Geometry: see drawing. Coordinates: mm, zero at the bounding-box minimum. A direction names the side the tool comes from. Coordinates: 2 decimals unless noted, no trailing zeros. Loops run counter-clockwise (first coordinate to the right, second up) from the corner with the lowest first, then second, coordinate; pieces in that order, holes last. Notation, with made-up numbers: (-27, -30) -> (18, -30) arc R10 cw to (18, -13) -> close; hole circle Ø6 at (43, 20.5). An arc over 180 degrees is marked (long way). Put each result on its own line as item: value. Start each with the question number.
1) Set-up query: the marked faces 1, 2 and 3. Return all of +Z, -Z, +X, -X, +Y, -Y with unobstructed straight access to the full face (end or side cutting, diameter ignored); none if empty.
2) Contact query for flat-ended pins moving along their axis: P1, Ø1, axis at x = 8.5, z = 7.5, coming from the -Y side; P2, Ø0.9, axis at x = 14.5, z = 4, coming from the -Y side; P3, Ø5, axis at x = 30, y = 10, coming from the -Z side. Output: stop coordinate, or through.
3) Cut plane A-A (x = 10). Return the cut outline in (y, z).
4) Cut plane C-C (x = 30). Return the cut outline in (y, z), plus the area to 3 significant figures.
5) Material intervals for L1, parallel to Y at x = 30, z = 3.75; L2, parallel to Y at x = 33, z = 1; L3, parallel to X at y = 30, z = 1.2, sorted ascending.
6) Pull-direction query (Z, two-part tool) for the marked faces 4, 5 and 6; classes: pulls with the +Z half, pulls with the -Z half, needs draft (parallel to the pull), parting line crosses it, or undercut.
7) Cut plane D-D (z = 1.25). Return the cut outline in (x, y), plus the area to 3 significant figures.
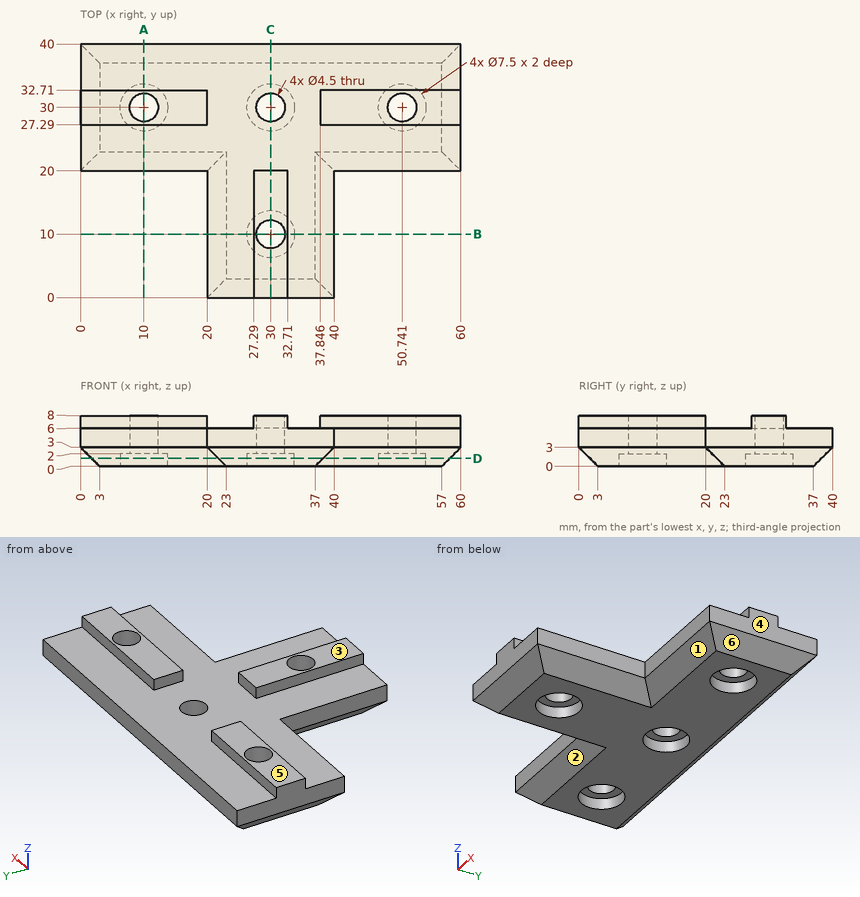
Results found:
1. face 1: -Z, +X, -Y
1. face 2: -Z, -X, -Y
1. face 3: +Z, +X, -X, +Y, -Y
2. P1: stops at y = 27.29
2. P2: stops at y = 20
2. P3: stops at z = 2
3. outline: (20, 3) -> (23, 0) -> (26.25, 0) -> (26.25, 2) -> (27.75, 2) -> (27.75, 8) -> (27.29, 8) -> (27.29, 6) -> (20, 6) -> close; (32.25, 2) -> (33.75, 2) -> (33.75, 0) -> (37, 0) -> (40, 3) -> (40, 6) -> (32.71, 6) -> (32.71, 8) -> (32.25, 8) -> close
4. outline: (0, 3) -> (3, 0) -> (6.25, 0) -> (6.25, 2) -> (7.75, 2) -> (7.75, 8) -> (0, 8) -> close; (12.25, 2) -> (13.75, 2) -> (13.75, 0) -> (26.25, 0) -> (26.25, 2) -> (27.75, 2) -> (27.75, 6) -> (20, 6) -> (20, 8) -> (12.25, 8) -> close; (32.25, 2) -> (33.75, 2) -> (33.75, 0) -> (37, 0) -> (40, 3) -> (40, 6) -> (32.25, 6) -> close
4. area: 196 mm2
5. L1: y = 0 to 7.75, 12.25 to 27.75, 32.25 to 40
5. L2: y = 2 to 7.75, 12.25 to 27.75, 32.25 to 38
5. L3: x = 1.8 to 6.25, 13.75 to 26.25, 33.75 to 46.99, 54.49 to 58.2
6. face 4: needs draft
6. face 5: pulls with the +Z half
6. face 6: pulls with the -Z half
7. outline: (1.75, 21.75) -> (21.75, 21.75) -> (21.75, 1.75) -> (38.25, 1.75) -> (38.25, 21.75) -> (58.25, 21.75) -> (58.25, 38.25) -> (1.75, 38.25) -> close; hole circle Ø7.5 at (10, 30); hole circle Ø7.5 at (30, 10); hole circle Ø7.5 at (30, 30); hole circle Ø7.5 at (50.74, 30)
7. area: 1,090 mm2
